Geometry: final body of the model. Coordinates: model frame, mm. Face numbers are marked on the shaded views. A direction names the side the tool comes from. Coordinates: 2 decimals unless noted, no trailing zeros. Write each loop counter-clockwise with the first axis right and the second up, starting at its lowest first coordinate (ties: lowest second). Pieces come first, ordered by that corner, then holes. Notation, with made-up numbers: (29.5, 54.5) - (63.5, 54.5) arc R18 cw to (63.5, 62.5) - close; hole circle Ø10 at (61, 57.5). An arc over 180 degrees is marked (long way). Answer as a JSON object with one key per item and string values. Group by question number.
Item 1: Section B-B on x = 478. Return loops of the section in (y, z), and give its area (3 significant figures).
Item 2: Set-up query: the marked faces 1 and 2. Return all of +Z, -Z, +X, -X, +Y, -Y with unobstructed straight access to the full face (end or side cutting, diameter ignored); none if empty.
Item 3: Line query: line 1 along Z through (x, y) = (471.5, 177); line 2 along X through (y, z) = (172, 0); line 3 along X through (y, z) = (202, 15). Output: solid intervals per line, ascending. Write a range as from..to.
Item 4: Section A-A on z = 0. Return loops of the section in (x, y), and give its area (3 significant figures).
Item 5: First-contact query: pin 1 Ø4 at (y, z) = (191.5, 29) entering from +X; pin 2 Ø4 at (y, z) = (187.5, 14.5) entering from +X; pin 3 Ø10 at (y, z) = (184.5, 26.5) entering from +X. Flat tips, straight axial feed; report the tip coordinate or a pass-through.
Item 6: Mould query, pull axis Z, two halves, no side actions, for the marked faces 3, 4 and 5. Classes: pulls with the +Z half, pulls with the -Z half, needs draft (parallel to the pull), parting line crosses it, or undercut.
Item 7: Section C-C on y = 201.5. Return loops of the section in (x, z).
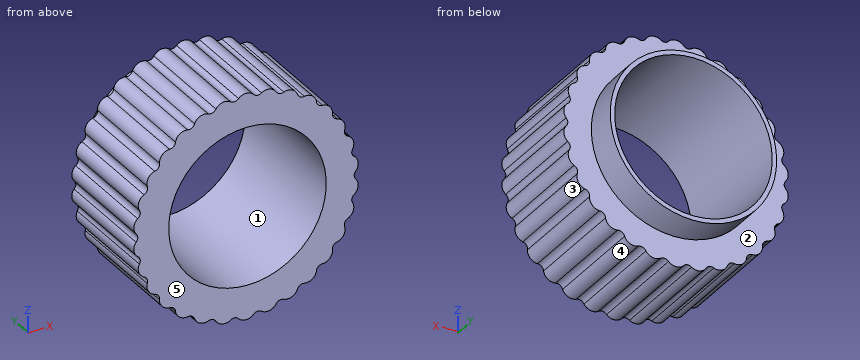
```python
from build123d import *

# Parameters (mm, degrees)
SKETCH7_R                = 27.493094195
BOSS_EXTRUDE2_DEPTH      = 36
BOSS_EXTRUDE3_DEPTH      = 11
BOSS_EXTRUDE3_DEPTH_BACK = 36
SKETCH8_R                = 27.992837321
SKETCH8_R_2              = 26.502402217


with BuildPart() as part:
    # Sketch7 → Boss-Extrude2 (new body)
    with BuildSketch(Plane(origin=(0, 195, 0), x_dir=(1, 0, 0), z_dir=(0, 1, 0))):
        with BuildLine():
            ThreePointArc((469.000007042, -36.915443923), (471.500007042, -37.950977828), (474.000007042, -36.915443923))
            ThreePointArc((474.000007042, -36.915443923), (475.305477345, -36.206631381), (476.729790403, -36.62853213))
            ThreePointArc((476.729790403, -36.62853213), (479.390459011, -37.121657908), (481.620528407, -35.588973676))
            ThreePointArc((481.620528407, -35.588973676), (482.750100638, -34.624227851), (484.231007137, -34.74077772))
            ThreePointArc((484.231007137, -34.74077772), (486.936060365, -34.669943408), (488.798734425, -32.707094505))
            ThreePointArc((488.798734425, -32.707094505), (489.703040856, -31.528579418), (491.175818076, -31.334684619))
            ThreePointArc((491.175818076, -31.334684619), (493.80703212, -30.702986016), (495.220903048, -28.395758358))
            ThreePointArc((495.220903048, -28.395758358), (495.86042115, -27.054980774), (497.260701657, -26.55911544))
            ThreePointArc((497.260701657, -26.55911544), (499.703079837, -25.394160806), (500.606354689, -22.843391312))
            ThreePointArc((500.606354689, -22.843391312), (500.953134452, -21.398949646), (502.219719271, -20.622785471))
            ThreePointArc((502.219719271, -20.622785471), (504.36651794, -18.975488914), (504.719719271, -16.292658452))
            ThreePointArc((504.719719271, -16.292658452), (504.758604755, -14.807681735), (505.836138051, -13.785140818))
            ThreePointArc((505.836138051, -13.785140818), (507.593531806, -11.727497102), (507.381223022, -9.029858236))
            ThreePointArc((507.381223022, -9.029858236), (507.110514745, -7.569247077), (507.951903142, -6.345019362))
            ThreePointArc((507.951903142, -6.345019362), (509.243085443, -3.966957392), (508.474545458, -1.372409886))
            ThreePointArc((508.474545458, -1.372409886), (507.906074671, 0), (508.474545458, 1.372409886))
            ThreePointArc((508.474545458, 1.372409886), (509.243085443, 3.966957392), (507.951903142, 6.345019362))
            ThreePointArc((507.951903142, 6.345019362), (507.110514745, 7.569247077), (507.381223022, 9.029858236))
            ThreePointArc((507.381223022, 9.029858236), (507.593531806, 11.727497102), (505.836138051, 13.785140818))
            ThreePointArc((505.836138051, 13.785140818), (504.758604755, 14.807681735), (504.719719271, 16.292658452))
            ThreePointArc((504.719719271, 16.292658452), (504.36651794, 18.975488914), (502.219719271, 20.622785471))
            ThreePointArc((502.219719271, 20.622785471), (500.953134452, 21.398949646), (500.606354689, 22.843391312))
            ThreePointArc((500.606354689, 22.843391312), (499.703079837, 25.394160806), (497.260701657, 26.55911544))
            ThreePointArc((497.260701657, 26.55911544), (495.86042115, 27.054980774), (495.220903048, 28.395758358))
            ThreePointArc((495.220903048, 28.395758358), (493.80703212, 30.702986016), (491.175818076, 31.334684619))
            ThreePointArc((491.175818076, 31.334684619), (489.703040856, 31.528579418), (488.798734425, 32.707094505))
            ThreePointArc((488.798734425, 32.707094505), (486.936060365, 34.669943408), (484.231007137, 34.74077772))
            ThreePointArc((484.231007137, 34.74077772), (482.750100638, 34.624227851), (481.620528407, 35.588973676))
            ThreePointArc((481.620528407, 35.588973676), (479.390459011, 37.121657908), (476.729790403, 36.62853213))
            ThreePointArc((476.729790403, 36.62853213), (475.305477345, 36.206631381), (474.000007042, 36.915443923))
            ThreePointArc((474.000007042, 36.915443923), (471.500007042, 37.950977828), (469.000007042, 36.915443923))
            ThreePointArc((469.000007042, 36.915443923), (467.694536739, 36.206631381), (466.270223681, 36.62853213))
            ThreePointArc((466.270223681, 36.62853213), (463.609555074, 37.121657908), (461.379485677, 35.588973676))
            ThreePointArc((461.379485677, 35.588973676), (460.249913446, 34.624227851), (458.769006947, 34.74077772))
            ThreePointArc((458.769006947, 34.74077772), (456.063953719, 34.669943408), (454.201279659, 32.707094505))
            ThreePointArc((454.201279659, 32.707094505), (453.296973228, 31.528579418), (451.824196008, 31.334684619))
            ThreePointArc((451.824196008, 31.334684619), (449.192981964, 30.702986016), (447.779111037, 28.395758358))
            ThreePointArc((447.779111037, 28.395758358), (447.139592935, 27.054980774), (445.739312427, 26.55911544))
            ThreePointArc((445.739312427, 26.55911544), (443.296934247, 25.394160806), (442.393659395, 22.843391312))
            ThreePointArc((442.393659395, 22.843391312), (442.046879632, 21.398949646), (440.780294813, 20.622785471))
            ThreePointArc((440.780294813, 20.622785471), (438.633496144, 18.975488914), (438.280294813, 16.292658452))
            ThreePointArc((438.280294813, 16.292658452), (438.241409329, 14.807681735), (437.163876034, 13.785140818))
            ThreePointArc((437.163876034, 13.785140818), (435.406482279, 11.727497102), (435.618791062, 9.029858236))
            ThreePointArc((435.618791062, 9.029858236), (435.889499339, 7.569247077), (435.048110942, 6.345019362))
            ThreePointArc((435.048110942, 6.345019362), (433.756928641, 3.966957392), (434.525468626, 1.372409886))
            ThreePointArc((434.525468626, 1.372409886), (435.093939413, 0), (434.525468626, -1.372409886))
            ThreePointArc((434.525468626, -1.372409886), (433.756928641, -3.966957392), (435.048110942, -6.345019362))
            ThreePointArc((435.048110942, -6.345019362), (435.889499339, -7.569247077), (435.618791062, -9.029858236))
            ThreePointArc((435.618791062, -9.029858236), (435.406482279, -11.727497102), (437.163876034, -13.785140818))
            ThreePointArc((437.163876034, -13.785140818), (438.241409329, -14.807681735), (438.280294813, -16.292658452))
            ThreePointArc((438.280294813, -16.292658452), (438.633496144, -18.975488914), (440.780294813, -20.622785471))
            ThreePointArc((440.780294813, -20.622785471), (442.046879632, -21.398949646), (442.393659395, -22.843391312))
            ThreePointArc((442.393659395, -22.843391312), (443.296934247, -25.394160806), (445.739312427, -26.55911544))
            ThreePointArc((445.739312427, -26.55911544), (447.139592935, -27.054980774), (447.779111037, -28.395758358))
            ThreePointArc((447.779111037, -28.395758358), (449.192981964, -30.702986016), (451.824196008, -31.334684619))
            ThreePointArc((451.824196008, -31.334684619), (453.296973228, -31.528579418), (454.201279659, -32.707094505))
            ThreePointArc((454.201279659, -32.707094505), (456.063953719, -34.669943408), (458.769006947, -34.74077772))
            ThreePointArc((458.769006947, -34.74077772), (460.249913446, -34.624227851), (461.379485677, -35.588973676))
            ThreePointArc((461.379485677, -35.588973676), (463.609555074, -37.121657908), (466.270223681, -36.62853213))
            ThreePointArc((466.270223681, -36.62853213), (467.694536739, -36.206631381), (469.000007042, -36.915443923))
        make_face()
        with Locations(Location((471.500007042, 0, 0), (0, 0, 270))):
            Circle(SKETCH7_R, mode=Mode.SUBTRACT)
    extrude(amount=-BOSS_EXTRUDE2_DEPTH)

    # Sketch8 → Boss-Extrude3 (add, two sides: drawn at the far end of the back side and taken through both)
    with BuildSketch(Plane(origin=(0, 195, 0), x_dir=(1, 0, 0), z_dir=(0, 1, 0)).offset(-BOSS_EXTRUDE3_DEPTH_BACK)):
        with Locations(Location((471.999750168, 0, 0), (0, 0, 270))):
            Circle(SKETCH8_R)
        with Locations(Location((471.999750168, 0, 0), (0, 0, 270))):
            Circle(SKETCH8_R_2, mode=Mode.SUBTRACT)
    extrude(amount=BOSS_EXTRUDE3_DEPTH + BOSS_EXTRUDE3_DEPTH_BACK)


solid = part.part
```
Checks:
{
 "1": {"outline": "(159, -37.14) - (195, -37.14) - (195, -27.34) - (206, -27.34) - (206, -25.81) - (159, -25.81) - close; (159, 25.81) - (206, 25.81) - (206, 27.34) - (195, 27.34) - (195, 37.14) - (159, 37.14) - close", "area": "849 mm^2"},
 "2": {"face 1": "+Y, -Y", "face 2": "+Y"},
 "3": {"line 1": "-37.95..-26.5, 26.5..37.95", "line 2": "435.09..445.5, 498.5..507.91", "line 3": "448.37..450.15, 493.85..495.63"},
 "4": {"outline": "(435.09, 159) - (445.5, 159) - (445.5, 206) - (444.01, 206) - (444.01, 195) - (435.09, 195) - close; (498.5, 159) - (507.91, 159) - (507.91, 195) - (499.99, 195) - (499.99, 206) - (498.5, 206) - close", "area": "746 mm^2"},
 "5": {"pin 1": "x = 495.92", "pin 2": "x = 507.23", "pin 3": "x = 500.88"},
 "6": {"face 3": "undercut", "face 4": "pulls with the -Z half", "face 5": "needs draft"},
 "7": {"outline": "circle Ø55.99 at (472, 0); hole circle Ø53 at (472, 0)"}
}
